Build history of the part. All positions in model axes, mm. A direction names the side the tool comes from. Round coordinates to 2 decimals unless told otherwise and drop trailing zeros. Loops run counter-clockwise (first coordinate to the right, second up) from the corner with the lowest first, then second, coordinate; pieces in that order, holes last. Notation, with made-up numbers: (61.5, -22.5) -> (105.5, -22.5) arc R9 cw to (105.5, -18.5) -> close; hole circle Ø3 at (43, 76.5). An arc over 180 degrees is marked (long way). Put each result on its own line as item: value. Start each with the question number.
Item 1: Drill centre lines: probe 1 along X at (y, z) = (3.7, -93.7); probe 2 along Z at (x, y) = (25.75, 4.05); probe 3 along X at (y, z) = (2.4, -93.7). Where is each one in solid material? Low to high. Write a range as [from, to].
Item 2: Flat gauge pins, fed straight in: pin 1 Ø4.5 at (x, z) = (25.5, -94.5) entering from +Y; pin 2 Ø3 at (x, z) = (25.46, -93.7) entering from -Y. Where does each tip first touch, or does it go through?
Item 3: Tool access for faces 1 (the flat face through (29.959, 3, -48)), 2 (the cylindrical face through (26.29, 3.91, -91.08)): list every direction of +Z, -Z, +X, -X, +Y, -Y with a clear straight run to the whole face (end or side of a thin tool).
Item 4: Pull direction X, two halves, no side cores. Call faces 3 (the flat face through (25, 2.9, -92)), 4 (the flat face through (22.7, 2.98, -0.91)), 5 (the flat face through (27, 3, -97.4)), 6 (the cylindrical face through (24.85, 1.72, -92.22)): +X half, -X half, draft (parallel to the pull), parting line (faces both ways), or undercut.
Item 5: Cut at A-A, the plane z = -93.7. List the corners of the cut face in (x, y).
```python
from build123d import *

# Parameters (mm, degrees)
SKETCH_1_W          = 8.2
SKETCH_1_H          = 97.4
EXTRUDE_1_DEPTH     = 5.4
SKETCH_2_R          = 1.6
CUT_EXTRUDE_1_DEPTH = 103.046451594
FILLET_1_R          = 0.5
FILLET_2_R          = 0.5
SKETCH_3_R          = 2.75
CUT_EXTRUDE_2_DEPTH = 2.5
FILLET_3_R          = 0.5


with BuildPart() as part:
    # 草图1 → 凸台-拉伸1 (new body)
    with BuildSketch(Plane(origin=(0, 0, 0), x_dir=(1, 0, 0), z_dir=(0, 1, 0))):
        with Locations((25.859277076, 48.7)):
            Rectangle(SKETCH_1_W, SKETCH_1_H)
    extrude(amount=EXTRUDE_1_DEPTH)

    # 草图2 → 切除-拉伸1 (cut, through all)
    with BuildSketch(Plane(origin=(0, 5.4, 0), x_dir=(1, 0, 0), z_dir=(0, 1, 0))):
        with Locations(Location((25.459277076, 93.7, 0), (0, 0, 270))):
            Circle(SKETCH_2_R)
        Polygon((21.759277076, 97.4), (23.609277076, 97.4), (21.759277076, 95.55), align=None)
        Polygon((21.759277076, 0), (23.609277076, 0), (21.759277076, 1.85), align=None)
    extrude(amount=-CUT_EXTRUDE_1_DEPTH, mode=Mode.SUBTRACT)

    # 圆角1
    fillet_1_edges = [part.edges().sort_by_distance(p)[0] for p in [
        (21.759277076, 0, -48.7),
        (26.784277076, 0, 0),
        (22.684277076, 0, -96.475),
        (22.684277076, 0, -0.925),
        (25.459277076, 0, -95.3),
        (26.784277076, 0, -97.4),
        (29.959277076, 0, -48.7),
    ]]
    fillet(fillet_1_edges, radius=FILLET_1_R)

    # 圆角2
    fillet_2_edges = [part.edges().sort_by_distance(p)[0] for p in [
        (29.959277076, 5.4, -48.7),
    ]]
    fillet(fillet_2_edges, radius=FILLET_2_R)

    # 草图3 → 切除-拉伸2 (cut)
    with BuildSketch(Plane(origin=(0, 5.4, 0), x_dir=(1, 0, 0), z_dir=(0, 1, 0))):
        with Locations(Location((25.459277076, 93.7, 0), (0, 0, 270))):
            Circle(SKETCH_3_R)
    extrude(amount=-CUT_EXTRUDE_2_DEPTH, mode=Mode.SUBTRACT)

    # 圆角3
    fillet_3_edges = [part.edges().sort_by_distance(p)[0] for p in [
        (25.459277076, 5.4, -96.45),
    ]]
    fillet(fillet_3_edges, radius=FILLET_3_R)


solid = part.part
```
Reply:
1. probe 1: x = [21.76, 22.71], [28.21, 29.96]
1. probe 2: z = [-97.4, -96.43], [-90.97, 0]
1. probe 3: x = [21.76, 23.86], [27.06, 29.96]
2. pin 1: stops at y = 5.36
2. pin 2: passes through
3. face 1: +Z, -Z, +X, +Y, -Y
3. face 2: +Y
4. face 3: undercut
4. face 4: -X half
4. face 5: draft
4. face 6: undercut
5. outline: (21.76, 0.5) arc R0.5 ccw to (22.26, 0) -> (23.36, 0) arc R0.5 ccw to (23.86, 0.5) -> (23.86, 2.9) -> (22.71, 2.9) -> (22.71, 4.9) arc R0.5 ccw to (22.21, 5.4) -> (21.76, 5.4) -> close; (27.06, 0.5) arc R0.5 ccw to (27.56, 0) -> (29.46, 0) arc R0.5 ccw to (29.96, 0.5) -> (29.96, 4.9) arc R0.5 ccw to (29.46, 5.4) -> (28.71, 5.4) arc R0.5 ccw to (28.21, 4.9) -> (28.21, 2.9) -> (27.06, 2.9) -> close
